Geometry: see drawing. Coordinates: mm, zero at the bounding-box minimum. A direction names the side the tool comes from. Coordinates: 2 decimals unless noted, no trailing zeros. Loops run counter-clockwise (first coordinate to the right, second up) from the corner with the lowest first, then second, coordinate; pieces in that order, holes last. Notation, with made-up numbers: (-12.75, 22) -> (41.25, 22) arc R21 ccw to (41.25, 53) -> close; hole circle Ø4 at (66.5, -29.5). An arc over 180 degrees is marked (long way). Put each result on its own line as item: value. Start each with the question number.
1) Cut plane A-A (z = 3.81). Return the cut outline in (x, y) (3 decimals).
2) Contact query for flat-ended pins moving along their axis: P1, Ø10, axis at x = 12, y = 11, coming from the +Z side; P2, Ø4, axis at y = 31.5, z = 3, coming from the -X side. Output: stop coordinate, or through.
3) Cut plane D-D (y = 23.5). Return the cut outline in (x, z).
4) Cut plane B-B (x = 7.62). Return the cut outline in (y, z) (3 decimals).
5) Material intervals for L1, parallel to Y at x = 2.75, z = 4 (3 decimals); L2, parallel to X at y = 12.5, z = 4.5, sorted ascending.
6) Set-up query: the marked faces 1 and 2. Return all of +Z, -Z, +X, -X, +Y, -Y with unobstructed straight access to the full face (end or side cutting, diameter ignored); none if empty.
7) Cut plane C-C (x = 2). Return the cut outline in (y, z) (3 decimals), plus the area to 3 significant figures.
8) Pull-direction query (Y, two-part tool) for the marked faces 3, 4 and 5; classes: pulls with the +Y half, pulls with the -Y half, needs draft (parallel to the pull), parting line crosses it, or undercut.
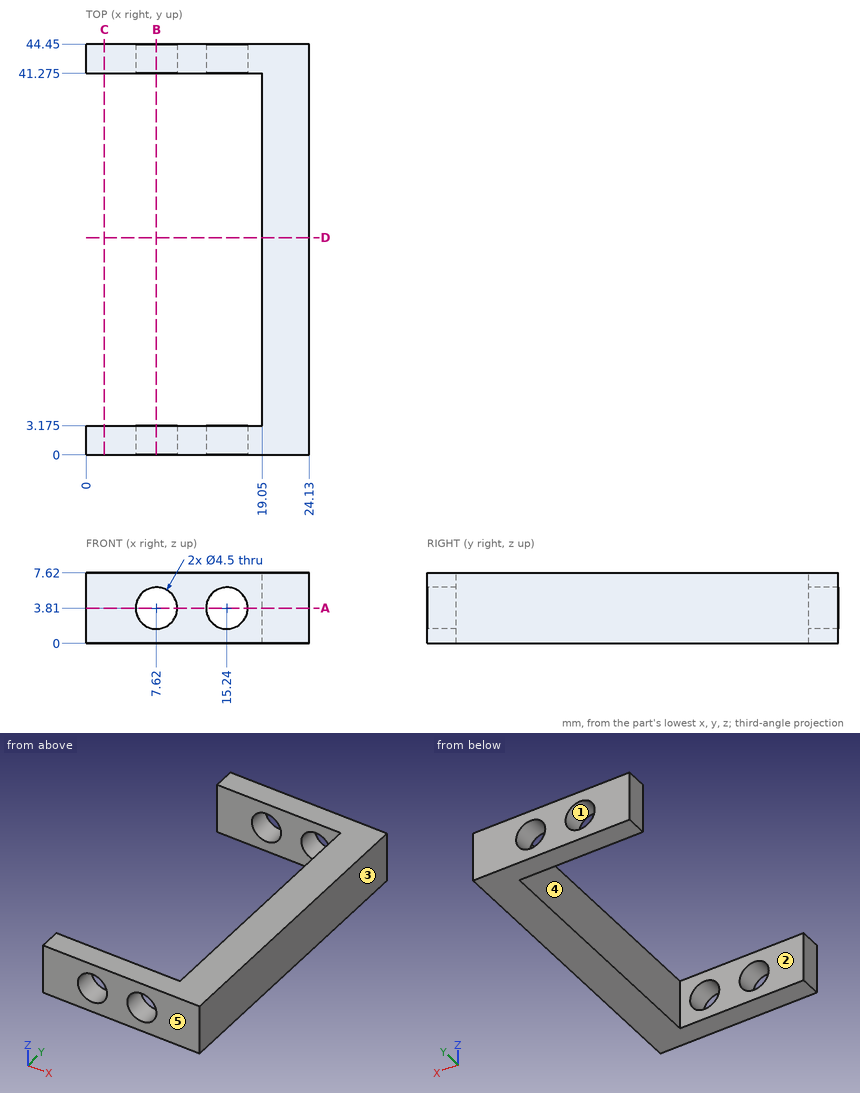
Results found:
1. outline: (0, 0) -> (5.37, 0) -> (5.37, 3.175) -> (0, 3.175) -> close; (0, 41.275) -> (5.37, 41.275) -> (5.37, 44.45) -> (0, 44.45) -> close; (9.87, 0) -> (12.99, 0) -> (12.99, 3.175) -> (9.87, 3.175) -> close; (9.87, 41.275) -> (12.99, 41.275) -> (12.99, 44.45) -> (9.87, 44.45) -> close; (17.49, 0) -> (24.13, 0) -> (24.13, 44.45) -> (17.49, 44.45) -> (17.49, 41.275) -> (19.05, 41.275) -> (19.05, 3.175) -> (17.49, 3.175) -> close
2. P1: passes through
2. P2: stops at x = 19.05
3. outline: (19.05, 0) -> (24.13, 0) -> (24.13, 7.62) -> (19.05, 7.62) -> close
4. outline: (0, 0) -> (3.175, 0) -> (3.175, 1.56) -> (0, 1.56) -> close; (0, 6.06) -> (3.175, 6.06) -> (3.175, 7.62) -> (0, 7.62) -> close; (41.275, 0) -> (44.45, 0) -> (44.45, 1.56) -> (41.275, 1.56) -> close; (41.275, 6.06) -> (44.45, 6.06) -> (44.45, 7.62) -> (41.275, 7.62) -> close
5. L1: y = 0 to 3.175, 41.275 to 44.45
5. L2: x = 19.05 to 24.13
6. face 1: +Y, -Y
6. face 2: +Z, -Z, -X
7. outline: (0, 0) -> (3.175, 0) -> (3.175, 7.62) -> (0, 7.62) -> close; (41.275, 0) -> (44.45, 0) -> (44.45, 7.62) -> (41.275, 7.62) -> close
7. area: 48.4 mm2
8. face 3: needs draft
8. face 4: undercut
8. face 5: pulls with the -Y half
